Work out the finished part from the listing and answer in its coordinate system (mm). Coordinates: 2 decimals unless noted, no trailing zeros. Write each loop counter-clockwise with the first axis right and the second up, starting at its lowest first coordinate (ties: lowest second). Pieces come first, ordered by that corner, then holes. Notation, with made-up numbers: (-13, 60) - (11, 60) arc R29 cw to (11, 91) - close; hole circle Ø3 at (65, 31). An arc over 180 degrees is marked (long way). Use one line per item in the form item = value. Start each with the question number.
Item 1: Given pin 1 (1 mm diameter, centred on x = 26, z = -13.5, fed in from -Y); pin 2 (0.9 mm diameter, centred on x = 60, y = 1.5, fed in from +Z); pin 3 (1.5 mm diameter, centred on x = 57, y = 1, fed in from -Z), each flat-ended and moving along its own axis, determine where each tip first touches the part or whether it passes through.
Item 2: A cutting plane is placed at A-A (z = 0.75). Write down the section's boundary in (x, y), then the cut area to 3 significant figures.
Item 3: A cutting plane is placed at B-B (x = 11.5). Write down the section's boundary in (y, z), then the cut area to 3 significant figures.
Item 4: Consider probe 1 along X at (y, z) = (0.5, -14); probe 2 along X at (y, z) = (1.45, -7); probe 3 along X at (y, z) = (1.9, -10.75). Determine where each line is inside the solid, lowest interval first.
Item 5: A cutting plane is placed at C-C (y = 1.65). Write down the section's boundary in (x, z).
Item 6: A cutting plane is placed at D-D (z = -12). Write down the section's boundary in (x, y), then the cut area to 3 significant figures.
from build123d import *

# Parameters (mm, degrees)
BOSS_EXTRUDE1_DEPTH = 3
SKETCH6_W           = 3
SKETCH6_H           = 7
CUT_EXTRUDE3_DEPTH  = 3
SKETCH7_R           = 1.5
CUT_EXTRUDE4_DEPTH  = 3
SKETCH8_W           = 3
SKETCH8_H           = 5
CUT_EXTRUDE5_DEPTH  = 3
SKETCH9_R           = 6
CUT_EXTRUDE6_DEPTH  = 3


with BuildPart() as part:
    # Sketch2 → Boss-Extrude1 (new body)
    with BuildSketch(Plane(origin=(0, 0, 0), x_dir=(1, 0, 0), z_dir=(0, 1, 0))):
        with BuildLine():
            Line((-3.583885407, 15.877073113), (62.416114593, 15.877073113))
            ThreePointArc((62.416114593, 15.877073113), (63.830328155, 15.291286675), (64.416114593, 13.877073113))
            Line((64.416114593, 13.877073113), (64.416114593, -0.122926887))
            ThreePointArc((64.416114593, -0.122926887), (63.830328155, -1.53714045), (62.416114593, -2.122926887))
            Line((62.416114593, -2.122926887), (-3.583885407, -2.122926887))
            ThreePointArc((-3.583885407, -2.122926887), (-4.99809897, -1.53714045), (-5.583885407, -0.122926887))
            Line((-5.583885407, -0.122926887), (-5.583885407, 13.877073113))
            ThreePointArc((-5.583885407, 13.877073113), (-4.99809897, 15.291286675), (-3.583885407, 15.877073113))
        make_face()
    extrude(amount=BOSS_EXTRUDE1_DEPTH)

    # Sketch6 → Cut-Extrude3 (cut)
    with BuildSketch(Plane(origin=(0, 3, 0), x_dir=(1, 0, 0), z_dir=(0, 1, 0))):
        with Locations((1.416114593, 12.377073113)):
            Rectangle(SKETCH6_W, SKETCH6_H)
        with Locations((57.416114593, 12.377073113)):
            Rectangle(SKETCH6_W, SKETCH6_H)
    extrude(amount=-CUT_EXTRUDE3_DEPTH, mode=Mode.SUBTRACT)

    # Sketch7 → Cut-Extrude4 (cut)
    with BuildSketch(Plane(origin=(0, 3, 0), x_dir=(1, 0, 0), z_dir=(0, 1, 0))):
        with Locations(Location((42.816114593, 6.977073113, 0), (0, 0, 270))):
            Circle(SKETCH7_R)
    extrude(amount=-CUT_EXTRUDE4_DEPTH, mode=Mode.SUBTRACT)

    # Sketch8 → Cut-Extrude5 (cut)
    with BuildSketch(Plane(origin=(0, 3, 0), x_dir=(1, 0, 0), z_dir=(0, 1, 0))):
        with Locations((60.416114593, 0.377073113)):
            Rectangle(SKETCH8_W, SKETCH8_H)
        with Locations((-1.583885407, 0.377073113)):
            Rectangle(SKETCH8_W, SKETCH8_H)
    extrude(amount=-CUT_EXTRUDE5_DEPTH, mode=Mode.SUBTRACT)

    # Sketch9 → Cut-Extrude6 (cut)
    with BuildSketch(Plane(origin=(0, 3, 0), x_dir=(1, 0, 0), z_dir=(0, 1, 0))):
        with Locations(Location((15.816114593, 6.877073113, 0), (0, 0, 270))):
            Circle(SKETCH9_R)
    extrude(amount=-CUT_EXTRUDE6_DEPTH, mode=Mode.SUBTRACT)


solid = part.part
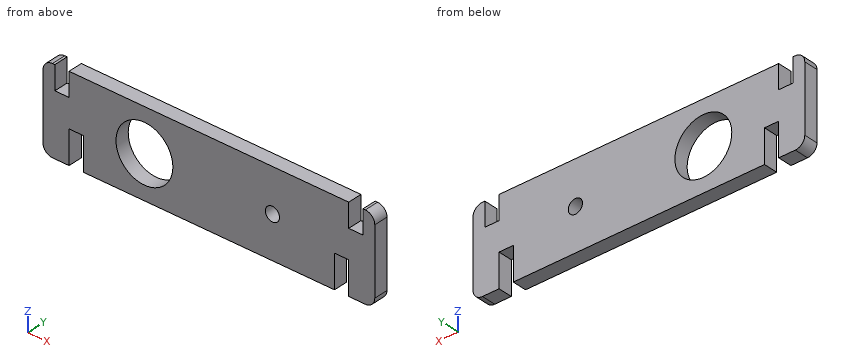
Answer:
q1.pin_1 = 0
q1.pin_2 = -2.88
q1.pin_3 = -8.88
q2.outline = (-5.48, 0) - (-3.08, 0) - (-3.08, 3) - (-5.48, 3) - close; (-0.08, 0) - (58.92, 0) - (58.92, 3) - (-0.08, 3) - close; (61.92, 0) - (64.32, 0) - (64.32, 3) - (61.92, 3) - close
q2.area = 191 mm²
q3.outline = (0, -15.88) - (3, -15.88) - (3, -11.04) - (0, -11.04) - close; (0, -2.71) - (3, -2.71) - (3, 2.12) - (0, 2.12) - close
q3.area = 29.0 mm²
q4.probe_1 = -5.58 to -0.08, 2.92 to 55.92, 58.92 to 64.41
q4.probe_2 = -5.58 to 9.82, 21.81 to 41.32, 44.32 to 64.42
q4.probe_3 = -5.58 to -0.08, 2.92 to 11.23, 20.4 to 55.92, 58.92 to 64.42
q5.outline = (-5.58, -13.88) arc R2 ccw to (-3.58, -15.88) - (-0.08, -15.88) - (-0.08, -8.88) - (2.92, -8.88) - (2.92, -15.88) - (55.92, -15.88) - (55.92, -8.88) - (58.92, -8.88) - (58.92, -15.88) - (62.42, -15.88) arc R2 ccw to (64.42, -13.88) - (64.42, 0.12) arc R2 ccw to (62.42, 2.12) - (61.92, 2.12) - (61.92, -2.88) - (58.92, -2.88) - (58.92, 2.12) - (-0.08, 2.12) - (-0.08, -2.88) - (-3.08, -2.88) - (-3.08, 2.12) - (-3.58, 2.12) arc R2 ccw to (-5.58, 0.12) - close; hole circle Ø12 at (15.82, -6.88); hole circle Ø3 at (42.82, -6.98)
q6.outline = (-5.58, 0) - (-0.08, 0) - (-0.08, 3) - (-5.58, 3) - close; (2.92, 0) - (12.69, 0) - (12.69, 3) - (2.92, 3) - close; (18.94, 0) - (55.92, 0) - (55.92, 3) - (18.94, 3) - close; (58.92, 0) - (64.42, 0) - (64.42, 3) - (58.92, 3) - close
q6.area = 173 mm²
